Can you work these out from the model? Positions are in its coordinate system, mm. Face numbers are marked on the shaded views. A direction names the side the tool comes from. Give positions to 0.01 mm unless a question says otherwise; leave off trailing zeros. Loops run counter-clockwise (first coordinate to the right, second up) from the corner with the lowest first, then second, coordinate; pieces in that order, holes last. Notation, with made-up numbers: (-13, 72) -> (8, 72) arc R16 ccw to (8, 91) -> close; hole circle Ø1 at (3, 62.25). An arc over 180 degrees is marked (long way). One line per question, with ' | ' between items.
from build123d import *

# Parameters (mm, degrees)
BOSS_EXTRUDE1_DEPTH     = 90
CUT_EXTRUDE6_DEPTH      = 115.405255561
CUT_EXTRUDE6_DEPTH_BACK = 44
SKETCH8_W               = 25
SKETCH8_H               = 15
CUT_EXTRUDE9_DEPTH      = 15
SKETCH13_W              = 16.5
SKETCH13_H              = 50
CUT_EXTRUDE18_DEPTH     = 11


with BuildPart() as part:
    # Sketch1 → Boss-Extrude1 (new body)
    with BuildSketch(Plane(origin=(0, 0, 0), x_dir=(1, 0, 0), z_dir=(0, 1, 0))):
        Polygon((0, 0), (70.5, 0), (70.5, 11), (64, 22), (44, 22), (44, 55.25), (0, 55.25), align=None)
    extrude(amount=BOSS_EXTRUDE1_DEPTH)

    # Sketch7 → Cut-Extrude6 (cut, two sides: drawn at the far end of the back side and taken through both)
    with BuildSketch(Plane(origin=(44, 0, 0), x_dir=(0, 0, -1), z_dir=(1, 0, 0)).offset(-CUT_EXTRUDE6_DEPTH_BACK)):
        with BuildLine():
            Line((243.604282259, 20), (55.25, 20))
            ThreePointArc((55.25, 20), (30.25, 45), (55.25, 70))
            Line((55.25, 70), (243.604282259, 70))
            Line((243.604282259, 70), (620.312846776, 70))
            Line((620.312846776, 70), (620.312846776, 20))
            Line((620.312846776, 20), (243.604282259, 20))
        make_face()
    extrude(amount=CUT_EXTRUDE6_DEPTH + CUT_EXTRUDE6_DEPTH_BACK, mode=Mode.SUBTRACT)

    # Sketch8 → Cut-Extrude9 (cut)
    with BuildSketch(Plane(origin=(0, 0, -55.25), x_dir=(-1, 0, 0), z_dir=(0, 0, -1))):
        with Locations((-22, 71)):
            Rectangle(SKETCH8_W, SKETCH8_H)
        with Locations((-22, 19)):
            Rectangle(SKETCH8_W, SKETCH8_H)
    extrude(amount=-CUT_EXTRUDE9_DEPTH, mode=Mode.SUBTRACT)

    # Sketch13 → Cut-Extrude18 (cut)
    with BuildSketch(Plane(origin=(0, 0, -22), x_dir=(-1, 0, 0), z_dir=(0, 0, -1))):
        with Locations((-62.25, 45)):
            Rectangle(SKETCH13_W, SKETCH13_H)
    extrude(amount=-CUT_EXTRUDE18_DEPTH, mode=Mode.SUBTRACT)


solid = part.part
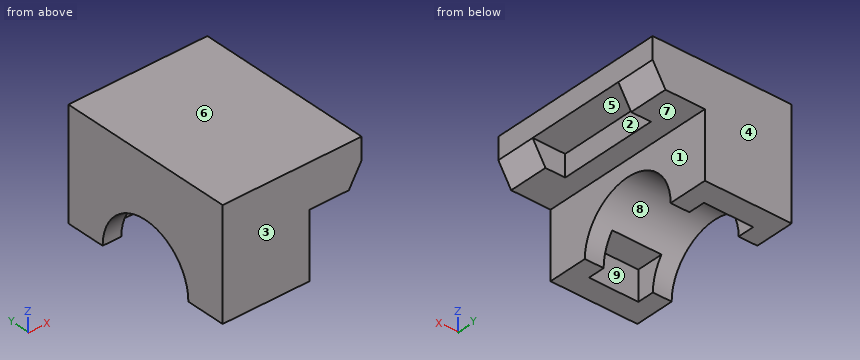
Q1. If we section it at C-C (y = 10): Write out the boundary of the cut face in (x, z).
Entries:
outline: (0, -55.25) -> (44, -55.25) -> (44, -22) -> (64, -22) -> (70.5, -11) -> (70.5, 0) -> (0, 0) -> close
Q2. On a 3-axis mill with a long thin cutter (end or side, diameter ignored), from which of +Z, -Z, +X, -X, +Y, -Y can I reach the whole of each face in a straight line? I mean the marked faces 5, 6, 7, 8 and 9. Say none if no direction works.
Entries:
face 5: -Z, +X | face 6: +Z, +X, -X, +Y, -Y | face 7: -Z, +X, +Y, -Y | face 8: -Z, +X, -X | face 9: -Z
Q3. If we section it at B-B (x = 62): Write out the boundary of the cut face in (y, z), plus the area to 3 significant figures.
Entries:
outline: (0, -22) -> (20, -22) -> (20, -11) -> (70, -11) -> (70, -22) -> (90, -22) -> (90, 0) -> (0, 0) -> close | area: 1,430 mm²
Q4. If we section it at D-D (z = -46): Write out the boundary of the cut face in (x, y), plus the area to 3 significant figures.
Entries:
outline: (0, 0) -> (44, 0) -> (44, 21.77) -> (34.5, 21.77) -> (34.5, 11.5) -> (9.5, 11.5) -> (9.5, 21.77) -> (0, 21.77) -> close; (0, 68.23) -> (9.5, 68.23) -> (9.5, 78.5) -> (34.5, 78.5) -> (34.5, 68.23) -> (44, 68.23) -> (44, 90) -> (0, 90) -> close | area: 1,400 mm²
Q5. If I drill on probe 1 along Y at (x, z) = (59.5, -18.5); probe 2 along Y at (x, z) = (17, -47.5); probe 3 along X at (y, z) = (76, -33.5), over which ranges is the centre line in solid material (lowest first)? Write a range as from..to.
Entries:
probe 1: 0..20, 70..90 | probe 2: 0..11.5, 78.5..90 | probe 3: 0..44
Q6. If we mould it in two halves opening along Y, with no side actions, what happens to the marked faces 1, 2, 3 and 4? For each: pulls with the +Y half, pulls with the -Y half, needs draft (parallel to the pull), parting line crosses it, or undercut.
Entries:
face 1: needs draft | face 2: undercut | face 3: pulls with the -Y half | face 4: pulls with the +Y half
Q7. For pin 1 Ø4 at (x, y) = (26, 19.5) entering from -Z; pin 2 Ø16.5 at (y, z) = (31.5, -41.5) entering from +X; pin 3 Ø18 at (x, y) = (65.5, 52) entering from -Z, each with a flat end and sliding along its axis, tell me the tip position at first contact or that it passes through.
Entries:
pin 1: z = -40.25 | pin 2: x = 44 | pin 3: z = -11
Q8. If we section it at A-A (z = -16.5): Write out the boundary of the cut face in (x, y).
Entries:
outline: (0, 0) -> (67.25, 0) -> (67.25, 20) -> (54, 20) -> (54, 70) -> (67.25, 70) -> (67.25, 90) -> (0, 90) -> close
